Can you work these out from the model? Positions are in its coordinate system, mm. A direction names the side the tool comes from. Give positions to 0.01 mm unless a question says otherwise; leave off trailing zeros. Order: outer loops, then holes, each group sorted by start corner. A loop starts at its lowest first (then second) coordinate and runs counter-clockwise, first axis right, second up.
Item 1: I want a section at C-C, the plane x = 48. Write out the boundary of the cut face in (y, z).
Item 2: If I drill on line 1 along Y through (x, z) = (31, 15.5); line 2 along X through (y, z) = (7, 11.75); line 3 along Z through (x, y) = (68, 12), over which ranges is the centre line in solid material (lowest first)?
Item 3: Which directions (+Z, -Z, +X, -X, +Y, -Y) give clear straight access to the entire face, cutting with the end or side of a thin tool? Please do faces 4 (the cylindrical face through (68.307, 5.151, 13.756)), 5 (the cylindrical face through (7.3, 30.84, 12.88)), 6 (the flat face through (57.719, 44, 16)), 7 (the cylindrical face through (3.131, 12.874, 8.735)).
Item 4: I want a section at A-A, the plane y = 19.7. Write out the boundary of the cut face in (x, z).
Item 5: If we mould it in two halves opening along X, with no side actions, what happens to faces 1 (the flat face through (24.719, 44, 16)), 2 (the flat face through (35, 35, 0)), 3 (the flat face through (0, 18, 13))? For each: +X half, -X half, draft (parallel to the pull), parting line (faces both ways), or undercut.
Item 6: I want a section at D-D, the plane z = 9.5. Count the separate pieces of the cut face and the enclosed holes in it, then the cut area to 3 significant figures.
Item 7: I want a section at B-B, the plane x = 39. Write out the boundary of the cut face in (y, z), then the cut area to 3 significant figures.
Item 8: I'm going to push flat-ended pins straight in: pin 1 Ø15.5 at (x, y) = (35.72, 44.45) entering from +Z; pin 2 Ø8 at (y, z) = (48, 4) entering from -X; pin 3 Ø1.4 at (y, z) = (5.7, 12.7) entering from +X; pin 4 Ø0.5 at (x, y) = (42, 35) entering from +Z. Where does each tip first touch, or does it pass through?
```python
from build123d import *

# Parameters (mm, degrees)
BOSS_EXTRUDE1_DEPTH     = 25.4
FILLET1_R               = 3.175
FILLET2_R               = 12.7
SKETCH3_R               = 1.190625
CUT_EXTRUDE1_DEPTH      = 6.35
CIRPATTERN1_COUNT       = 4
SKETCH4_R               = 3.96875
CUT_EXTRUDE2_DEPTH      = 6.35
SKETCH5_R               = 3.175
CUT_EXTRUDE3_DEPTH      = 25.4
SKETCH6_W               = 24
SKETCH6_H               = 12
CUT_EXTRUDE4_DEPTH      = 23
SKETCH7_W               = 5
SKETCH7_H               = 12
SKETCH7_W_2             = 4
CUT_EXTRUDE5_DEPTH      = 19
FILLET6_R               = 0.396875
CUT_EXTRUDE6_DEPTH      = 95.331537177
CUT_EXTRUDE6_DEPTH_BACK = 4
SKETCH9_W               = 9.525
SKETCH9_H               = 15.875
CUT_EXTRUDE7_DEPTH      = 25.4
FILLET7_DEPTH           = 25.4
FILLET7_2_DEPTH         = 25.4
FILLET8_R               = 12.7
SKETCH10_R              = 0.79375
CUT_EXTRUDE8_DEPTH      = 12.7


with BuildPart() as part:
    # Sketch2 → Boss-Extrude1 (new body)
    with BuildSketch(Plane.XY):
        Polygon((0, 0), (0, 57.15), (71.4375, 57.15), (71.4375, 0), (65.0875, 0), (65.0875, 31.75), (6.35, 31.75), (6.35, 0), align=None)
    extrude(amount=BOSS_EXTRUDE1_DEPTH)

    # Fillet1
    fillet1_edges = [part.edges().sort_by_distance(p)[0] for p in [
        (65.0875, 31.75, 12.7),
        (6.35, 31.75, 12.7),
    ]]
    fillet(fillet1_edges, radius=FILLET1_R)

    # Fillet2
    fillet2_edges = [part.edges().sort_by_distance(p)[0] for p in [
        (3.175, 0, 0),
        (68.2625, 0, 0),
        (3.175, 0, 25.4),
        (68.2625, 0, 25.4),
    ]]
    fillet(fillet2_edges, radius=FILLET2_R - 0.0001)  # a hair under: the kernel refuses the full size

    # Sketch3 → Cut-Extrude1 (cut)
    with BuildSketch(Plane(origin=(71.4375, 0, 0), x_dir=(0, 0, -1), z_dir=(1, 0, 0))):
        with Locations(Location((-12.7, 19.7, 0), (0, 0, 90))):
            Circle(SKETCH3_R)
    cut_extrude1 = extrude(amount=-CUT_EXTRUDE1_DEPTH, mode=Mode.SUBTRACT)

    # CirPattern1: Cut-Extrude1 ×4 about axis
    cirpattern1_axis = Axis((0, 12.7, 12.7), (1, 0, 0))
    for i in range(1, CIRPATTERN1_COUNT):
        add(cut_extrude1.rotate(cirpattern1_axis, i * 360 / CIRPATTERN1_COUNT), mode=Mode.SUBTRACT)

    # Sketch4 → Cut-Extrude2 (cut)
    with BuildSketch(Plane.ZY):
        with Locations((12.7, 12.7)):
            Circle(SKETCH4_R)
    extrude(amount=-CUT_EXTRUDE2_DEPTH, mode=Mode.SUBTRACT)

    # Sketch5 → Cut-Extrude3 (cut)
    with BuildSketch(Plane.XY.offset(25.4)):
        with Locations((35.71875, 44.45)):
            Circle(SKETCH5_R)
    extrude(amount=-CUT_EXTRUDE3_DEPTH, mode=Mode.SUBTRACT)

    # Sketch6 → Cut-Extrude4 (cut)
    with BuildSketch(Plane.XY.offset(25.4)):
        with Locations((41.71875, 44.45)):
            Rectangle(SKETCH6_W, SKETCH6_H)
    extrude(amount=-CUT_EXTRUDE4_DEPTH, mode=Mode.SUBTRACT)

    # Sketch7 → Cut-Extrude5 (cut)
    with BuildSketch(Plane.XY.offset(25.4)):
        with Locations((27.21875, 44.45)):
            Rectangle(SKETCH7_W, SKETCH7_H)
        with Locations((55.71875, 44.45)):
            Rectangle(SKETCH7_W_2, SKETCH7_H)
    extrude(amount=-CUT_EXTRUDE5_DEPTH, mode=Mode.SUBTRACT)

    # Fillet6
    fillet6_edges = [part.edges().sort_by_distance(p)[0] for p in [
        (24.71875, 44.45, 6.4),
        (57.71875, 44.45, 6.4),
        (53.71875, 44.45, 2.4),
        (29.71875, 44.45, 2.4),
    ]]
    fillet(fillet6_edges, radius=FILLET6_R)

    # Sketch8 → Cut-Extrude6 (cut, two sides: drawn at the far end of the back side and taken through both)
    with BuildSketch(Plane.XY.offset(2.4).offset(-CUT_EXTRUDE6_DEPTH_BACK)):
        with BuildLine():
            Line((42.71875, 47.7), (40.76231025, 47.7))
            ThreePointArc((40.76231025, 47.7), (29.71875, 44.45), (40.76231025, 41.2))
            Line((40.76231025, 41.2), (42.71875, 41.2))
            ThreePointArc((42.71875, 41.2), (45.96875, 44.45), (42.71875, 47.7))
        make_face()
    extrude(amount=CUT_EXTRUDE6_DEPTH + CUT_EXTRUDE6_DEPTH_BACK, mode=Mode.SUBTRACT)

    # Sketch9 → Cut-Extrude7 (cut)
    with BuildSketch(Plane.XY.offset(25.4)):
        with Locations((4.7625, 49.2125)):
            Rectangle(SKETCH9_W, SKETCH9_H)
        with Locations((66.675, 49.2125)):
            Rectangle(SKETCH9_W, SKETCH9_H)
    extrude(amount=-CUT_EXTRUDE7_DEPTH, mode=Mode.SUBTRACT)

    # Fillet7: read off the stored shape, not the designer's step
    # Fillet7 outline → Fillet7 (cut)
    with BuildSketch(Plane.XY):
        with BuildLine():
            ThreePointArc((66.675, 41.275), (70.042596045, 39.880096045), (71.4375, 36.5125))
            Line((71.4375, 36.5125), (71.4375, 41.275))
            Line((71.4375, 41.275), (66.675, 41.275))
        make_face()
        with BuildLine():
            ThreePointArc((0, 36.5125), (1.394903955, 39.880096045), (4.7625, 41.275))
            Line((4.7625, 41.275), (0, 41.275))
            Line((0, 41.275), (0, 36.5125))
        make_face()
    extrude(amount=FILLET7_DEPTH, mode=Mode.SUBTRACT)

    # Fillet7 2 outline → Fillet7 2 (add)
    with BuildSketch(Plane.XY):
        with BuildLine():
            Line((61.9125, 41.275), (66.675, 41.275))
            ThreePointArc((66.675, 41.275), (63.307403955, 42.669903955), (61.9125, 46.0375))
            Line((61.9125, 46.0375), (61.9125, 41.275))
        make_face()
        with BuildLine():
            ThreePointArc((9.525, 46.0375), (8.130096045, 42.669903955), (4.7625, 41.275))
            Line((4.7625, 41.275), (9.525, 41.275))
            Line((9.525, 41.275), (9.525, 46.0375))
        make_face()
    extrude(amount=FILLET7_2_DEPTH)

    # Fillet8
    fillet8_edges = [part.edges().sort_by_distance(p)[0] for p in [
        (9.525, 57.15, 12.7),
        (61.9125, 57.15, 12.7),
    ]]
    fillet(fillet8_edges, radius=FILLET8_R)

    # Sketch10 → Cut-Extrude8 (cut)
    with BuildSketch(Plane.XY.offset(25.4)):
        with Locations((29.36875, 53.975)):
            Circle(SKETCH10_R)
        with Locations((42.06875, 53.975)):
            Circle(SKETCH10_R)
        with Locations((29.36875, 34.925)):
            Circle(SKETCH10_R)
        with Locations((42.06875, 34.925)):
            Circle(SKETCH10_R)
    extrude(amount=-CUT_EXTRUDE8_DEPTH, mode=Mode.SUBTRACT)


solid = part.part
```
Results list:
1. outline: (31.75, 0) - (57.15, 0) - (57.15, 25.4) - (50.45, 25.4) - (50.45, 2.4) - (38.45, 2.4) - (38.45, 25.4) - (31.75, 25.4) - close
2. line 1: y = 31.75 to 38.45, 50.45 to 57.15
2. line 2: x = 0 to 6.35, 65.09 to 71.44
2. line 3: z = 0.02 to 4.74, 6.66 to 18.74, 20.66 to 25.38
3. face 4: +X
3. face 5: +Z, -Z, -Y
3. face 6: +Z
3. face 7: -X
4. outline: (0, 0) - (6.35, 0) - (6.35, 25.4) - (0, 25.4) - close; (65.09, 0) - (71.44, 0) - (71.44, 11.51) - (65.09, 11.51) - close; (65.09, 13.89) - (71.44, 13.89) - (71.44, 25.4) - (65.09, 25.4) - close
5. face 1: undercut
5. face 2: draft
5. face 3: -X half
6. separate pieces: 2
6. enclosed holes: 1
6. area: 1,420 mm2
7. outline: (31.75, 0) - (39.43, 0) - (39.43, 2.4) - (38.45, 2.4) - (38.45, 25.4) - (31.75, 25.4) - close; (49.47, 0) - (57.15, 0) - (57.15, 25.4) - (50.45, 25.4) - (50.45, 2.4) - (49.47, 2.4) - close
7. area: 345 mm2
8. pin 1: stops at z = 25.4
8. pin 2: stops at x = 9.07
8. pin 3: stops at x = 6.35
8. pin 4: stops at z = 12.7
